Design review of the part shown in the three views and the two pictorial views. Dimensions are in mm from the part's minimum x, y and z. A direction names the side the tool comes from. Give positions to 0.01 mm unless a question says otherwise; leave off trailing zeros. Loops run counter-clockwise (first coordinate to the right, second up) from the corner with the lowest first, then second, coordinate; pieces in that order, holes last. Notation, with made-up numbers: (-25, 65.25) -> (19, 65.25) arc R15 cw to (19, 80.25) -> close; hole circle Ø8 at (24.25, -19). An arc over 180 degrees is marked (long way). Answer as CSV lines item,"result".
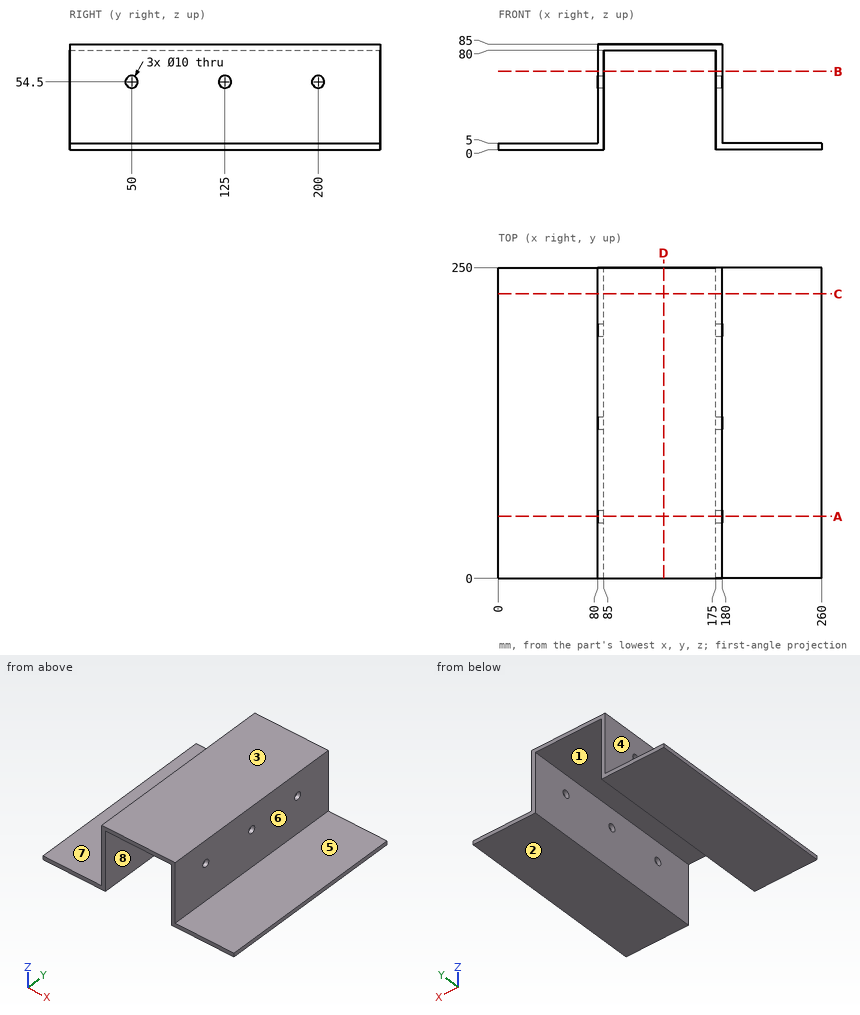
Q1. For the marked faces 1, 2, 3, 4 and 5, list the 3-axis set-ups (+Z, -Z, +X, -X, +Y, -Y) from which the entire face can be reached by the end or side of a thin tool; tool diameter is ignored.
Filled sheet:
face 1,"-Z, +Y, -Y"
face 2,"-Z, +X, -X, +Y, -Y"
face 3,"+Z, +X, -X, +Y, -Y"
face 4,"+Z, -X, +Y, -Y"
face 5,"+Z, +X, +Y, -Y"
Q2. The part is to be moulded in two halves that separate along X. For the marked faces 6, 7 and 8, say which applies: pulls with the +X half, pulls with the -X half, needs draft (parallel to the pull), parting line crosses it, or undercut.
Filled sheet:
face 6,"pulls with the +X half"
face 7,"needs draft"
face 8,"undercut"
Q3. Clearance check with flat-ended pins moving along their axes: pin 1 Ø13 at (y, z) = (50, 54.5) entering from +X; pin 2 Ø12 at (y, z) = (157, 43) entering from -X; pin 3 Ø3 at (x, y) = (103, 211) entering from -Z. State where each tip first meets the part, or that it passes through.
Filled sheet:
pin 1,"stops at x = 180"
pin 2,"stops at x = 80"
pin 3,"stops at z = 80"
Q4. We need section A-A, the plane y = 50. State the section outline as (x, z) points.
Filled sheet:
outline,"(0, 0) -> (85, 0) -> (85, 49.5) -> (80, 49.5) -> (80, 5) -> (0, 5) -> close; (80, 59.5) -> (85, 59.5) -> (85, 80) -> (175, 80) -> (175, 59.5) -> (180, 59.5) -> (180, 85) -> (80, 85) -> close; (175, 0) -> (260, 0) -> (260, 5) -> (180, 5) -> (180, 49.5) -> (175, 49.5) -> close"
Q5. We need section B-B, the plane z = 63. State the section outline as (x, y) points, and give its area (3 significant figures).
Filled sheet:
outline,"(80, 0) -> (85, 0) -> (85, 250) -> (80, 250) -> close; (175, 0) -> (180, 0) -> (180, 250) -> (175, 250) -> close"
area,"2,500 mm^2"
Q6. To check wall thickness, follow probe 1 along Y at (x, z) = (176.15, 54.5); probe 2 along X at (y, z) = (170.5, 6.5); probe 3 along Z at (x, y) = (240, 198.5). State the ranges of each line that lie inside material, in increasing order. Write a range as from..to.
Filled sheet:
probe 1,"y = 0..45, 55..120, 130..195, 205..250"
probe 2,"x = 80..85, 175..180"
probe 3,"z = 0..5"
Q7. We need section C-C, the plane y = 229. State the section outline as (x, z) points.
Filled sheet:
outline,"(0, 0) -> (85, 0) -> (85, 80) -> (175, 80) -> (175, 0) -> (260, 0) -> (260, 5) -> (180, 5) -> (180, 85) -> (80, 85) -> (80, 5) -> (0, 5) -> close"
Q8. We need section D-D, the plane x = 133. State the section outline as (y, z) points.
Filled sheet:
outline,"(0, 80) -> (250, 80) -> (250, 85) -> (0, 85) -> close"
